The listing builds one solid part. Answer for the finished solid, in the listing's coordinates (mm). A direction names the side the tool comes from. Give positions to 0.01 mm unless a question says otherwise; leave off trailing zeros. Order: outer loops, then holes, each group sorted by start corner. A loop starts at its lowest first (then second) coordinate and runs counter-clockwise, first axis right, second up. Notation, with made-up numbers: (-21.5, 19.25) -> (15.5, 19.25) arc R34 ccw to (15.5, 51.25) -> close; hole circle Ø8 at (51, 15.25). An arc over 180 degrees is marked (long way). Answer as a JSON object with one key per item and string values. Group by question number.
Autodesk Inventor part; units mm, degrees
ref_plane "YZ Plane" through (0, 0, 0) normal (1, 0, 0) x (0, 1, 0)
ref_plane "XZ Plane" through (0, 0, 0) normal (0, 1, 0) x (-1, 0, 0)
ref_plane "XY Plane" through (0, 0, 0) normal (0, 0, 1) x (1, 0, 0)
sketch "Sketch1" plane through (0, 0, 0) normal (0, 1, 0) x (-1, 0, 0)
  line L0 (-7.5, 5.5) -> (7.5, 5.5)
  line L1 (7.5, 5.5) -> (7.5, -5.5)
  line L2 (7.5, -5.5) -> (-7.5, -5.5)
  line L3 (-7.5, -5.5) -> (-7.5, 5.5)
  line L4 (-7.5, 5.5) -> (7.5, -5.5) construction
  line L5 (7.5, 5.5) -> (-7.5, -5.5) construction
  circle A0 centre (0, -5.5) radius 7.5 construction
  arc A1 (-7.5, -5.5) -> (7.5, -5.5) centre (0, -5.5) ccw
  point P0 (0, 0)
  dimension "d0" = 11
  dimension "d1" = 15
extrude "Extrusion1" add sketch "Sketch1" along normal blind 8
sketch "Sketch2" plane through (0, 0, 0) normal (0, -1, 0) x (1, 0, 0)
  line L0 (7.5, 9.25) -> (-7.5, 9.25)
  line L1 (-7.5, 9.25) -> (-7.5, -20.75)
  line L2 (-7.5, -20.75) -> (7.5, -20.75)
  line L3 (7.5, -20.75) -> (7.5, 9.25)
  line L4 (7.5, 9.25) -> (-7.5, -20.75) construction
  line L5 (-7.5, 9.25) -> (7.5, -20.75) construction
  line L6 (-7.5, 5.5) -> (7.5, 5.5)
  line L7 (7, 8.75) -> (-7, 8.75) construction
  line L8 (-7, 8.75) -> (-7, -20.25) construction
  line L9 (-7, -20.25) -> (7, -20.25) construction
  line L10 (7, -20.25) -> (7, 8.75) construction
  line L11 (7, 8.75) -> (-7, -20.25) construction
  line L12 (-7, 8.75) -> (7, -20.25) construction
  point P0 (0, 0)
  point P1 (0, -5.75)
  dimension "d4" = 15
  dimension "d5" = 30
  dimension "d6" = 3.75
  dimension "d18" = 0.5
  dimension "d19" = 0.5
sketch "Sketch4" plane through (0, 0, 0) normal (0, -1, 0) x (1, 0, 0)
  line L0 (-7.5, -5.5) -> (-7.5, 5.5)
  line L1 (-7.5, 3.75) -> (-6.5, 3.75)
  line L2 (-6.5, 3.75) -> (-6.5, 0.75)
  line L3 (-6.5, 0.75) -> (-7.5, 0.75)
  line L4 (-7.5, 0.75) -> (-7.5, 3.75)
  line L5 (7.5, 5.5) -> (7.5, -5.5)
  line L6 (7.5, 0.75) -> (6.5, 0.75)
  line L7 (6.5, 0.75) -> (6.5, 3.75)
  line L8 (6.5, 3.75) -> (7.5, 3.75)
  line L9 (7.5, 3.75) -> (7.5, 0.75)
  line L10 (-7.5, -20.25) -> (7.5, -20.25) construction
  line L11 (7.5, -20.25) -> (7.5, 9.75) construction
  line L12 (7.5, 9.75) -> (-7.5, 9.75) construction
  line L13 (-7.5, 9.75) -> (-7.5, -20.25) construction
  line L14 (-7.5, -20.25) -> (7.5, 9.75) construction
  line L15 (7.5, -20.25) -> (-7.5, 9.75) construction
  line L16 (-7.5, 5.5) -> (7.5, 5.5) construction
  arc A0 (-7.5, -5.5) -> (7.5, -5.5) centre (0, -5.5) ccw construction
  point P0 (0, 0)
  point P1 (0, -5.25)
  point P2 (0, -13)
  point P3 (-7, 3.75)
  point P4 (-7.5, 0.75)
  point P5 (-7, 0.75)
  point P6 (7.5, 3.75)
  point P7 (-7.5, 0.75)
  dimension "d20" = 1
  dimension "d21" = 3
  dimension "d22" = 1
  dimension "d23" = 3
  dimension "d24" = 15
  dimension "d25" = 30
  dimension "d27" = 7.25
  dimension "d106" = 0.75
extrude "Extrusion3" add sketch "Sketch4" along normal blind 1.6
sketch "Sketch6" plane through (0, 0, 0) normal (0, -1, 0) x (1, 0, 0)
  line L0 (7.5, 11.25) -> (-7.5, 11.25)
  line L1 (-7.5, 11.25) -> (-7.5, -18.75)
  line L2 (-7.5, -18.75) -> (7.5, -18.75)
  line L3 (7.5, -18.75) -> (7.5, 11.25)
  line L4 (7.5, 11.25) -> (-7.5, -18.75) construction
  line L5 (-7.5, 11.25) -> (7.5, -18.75) construction
  line L6 (7, 10.75) -> (-7, 10.75) construction
  line L7 (-7, 10.75) -> (-7, -18.25) construction
  line L8 (-7, -18.25) -> (7, -18.25) construction
  line L9 (7, -18.25) -> (7, 10.75) construction
  line L10 (7, 10.75) -> (-7, -18.25) construction
  line L11 (-7, 10.75) -> (7, -18.25) construction
  circle A0 centre (0, -3.75) radius 1
  circle A1 centre (0, -3.75) radius 1.5
  line L12 (-6.5, 4.5) -> (6.5, 4.5)
  line L13 (6.5, 4.5) -> (6.5, -5.5)
  line L14 (6.5, -5.5) -> (-6.5, -5.5)
  line L15 (-6.5, -5.5) -> (-6.5, 4.5)
  line L16 (-7.5, 5.5) -> (7.5, 5.5)
  arc A2 (-7.5, -5.5) -> (7.5, -5.5) centre (0, -5.5) ccw
  circle A3 centre (0, -5.5) radius 6.5
  point P0 (0, 0)
  point P1 (-7.5, -3.75)
  point P2 (6.5, -5.5)
  dimension "d31" = 15
  dimension "d32" = 30
  dimension "d34" = 0.5
  dimension "d35" = 0.5
  dimension "d36" = 2
  dimension "d37" = 0.5
  dimension "d38" = 1
  dimension "d39" = 1
  dimension "d40" = 1
  dimension "d41" = 1
  dimension "d107" = 3.75
extrude "Extrusion4" cut sketch "Sketch6" against normal blind 2.5 contours A0 | L12 L13 A3 L15 | A3 L14 | L14 A3
sketch "Sketch10" plane through (0, 8, 0) normal (0, 1, 0) x (1, 0, 0)
  point P0 (0, 0)
sketch "Sketch11" plane through (0, 0, 0) normal (0, -1, 0) x (1, 0, 0)
  line L0 (-5, 3.5) -> (-2.5, 3.5)
  line L1 (-2.5, 3.5) -> (-2.5, 2)
  line L2 (-2.5, 2) -> (-5, 2)
  line L3 (-5, 2) -> (-5, 3.5)
  line L4 (2.5, 3.5) -> (5, 3.5)
  line L5 (5, 3.5) -> (5, 2)
  line L6 (5, 2) -> (2.5, 2)
  line L7 (2.5, 2) -> (2.5, 3.5)
  line L8 (-6.5, 3.75) -> (-7.5, 3.75)
  line L9 (-6.5, 0.75) -> (-6.5, 3.75)
  line L10 (6.5, 3.75) -> (6.5, 0.75)
  line L11 (-6.5, 4.5) -> (6.5, 4.5)
  line L12 (-1.25, -11) -> (1.25, -11)
  line L13 (1.25, -11) -> (1.25, -9.5)
  line L14 (1.25, -9.5) -> (-1.25, -9.5)
  line L15 (-1.25, -9.5) -> (-1.25, -11)
  circle A0 centre (0, -3.75) radius 1
  point P0 (0, 0)
  point P1 (-3.75, 3.5)
  point P2 (3.75, 3.5)
  point P3 (1.25, -10.25)
  point P4 (2.5, 2.75)
  point P5 (0, -9.5)
  point P6 (3.75, 2)
  point P7 (-2.5, 2.75)
  dimension "d51" = 2.5
  dimension "d52" = 1.5
  dimension "d55" = 2.75
  dimension "d56" = 2.75
  dimension "d60" = 13
  dimension "d61" = 3.75
  dimension "d62" = 3.75
  dimension "d103" = 6.5
  dimension "d104" = 6.5
extrude "Extrusion8" cut sketch "Sketch11" against normal blind 10 contours L0 L1 L2 L3 | L4 L5 L6 L7 | L15 L14 L13 L12
sketch "Sketch12" plane through (0, 2.5, 0) normal (0, -1, 0) x (1, 0, 0)
  line L0 (5, 2) -> (5, 3.5) construction
  line L1 (2.5, 2) -> (5, 2) construction
  line L2 (5, 3.5) -> (2.5, 3.5) construction
  line L3 (2.5, 3.5) -> (2.5, 2) construction
  line L4 (2.5, 2) -> (5, 2) construction
  line L5 (5, 2) -> (5, 3.5) construction
  line L6 (-2.5, 2) -> (-2.5, 3.5) construction
  line L7 (-2.5, 2) -> (-5, 2) construction
  line L8 (-2.5, 3.5) -> (-5, 3.5) construction
  line L9 (-5, 3.5) -> (-5, 2) construction
  line L10 (-5, 2) -> (-2.5, 2) construction
  line L11 (-2.5, 2) -> (-2.5, 3.5) construction
  line L12 (-1.25, -9.5) -> (1.25, -9.5) construction
  line L13 (-1.25, -9.5) -> (-1.25, -11) construction
  line L14 (1.25, -9.5) -> (-1.25, -9.5) construction
  line L15 (-1.25, -9.5) -> (-1.25, -11) construction
  line L16 (-1.25, -11) -> (1.25, -11) construction
  line L17 (1.25, -11) -> (1.25, -9.5) construction
  line L18 (5.5, 3.5) -> (2, 3.5)
  line L19 (2, 3.5) -> (2, 2)
  line L20 (2, 2) -> (5.5, 2)
  line L21 (5.5, 2) -> (5.5, 3.5)
  line L22 (1.75, -9.5) -> (-1.75, -9.5)
  line L23 (-1.75, -9.5) -> (-1.75, -11)
  line L24 (-1.75, -11) -> (1.75, -11)
  line L25 (1.75, -11) -> (1.75, -9.5)
  line L26 (-2, 3.5) -> (-5.5, 3.5)
  line L27 (-5.5, 3.5) -> (-5.5, 2)
  line L28 (-5.5, 2) -> (-2, 2)
  line L29 (-2, 2) -> (-2, 3.5)
  point P0 (0, 0)
  point P1 (-2.5, 2.75)
  point P2 (-2, 2.75)
  point P3 (-3.75, 2)
  point P4 (-3.75, 2)
  point P5 (-3.75, 3.5)
  point P6 (-3.75, 3.5)
  point P7 (-5, 2.75)
  point P8 (-5.5, 2.75)
  point P9 (1.25, -10.25)
  point P10 (1.75, -10.25)
  point P11 (0, -11)
  point P12 (-1.25, -10.25)
  dimension "d63" = 0.5
  dimension "d64" = 0
  dimension "d65" = 0
  dimension "d67" = 0.5
  dimension "d68" = 0
  dimension "d69" = 0
  dimension "d70" = 0.5
  dimension "d71" = 0.5
  dimension "d72" = 0
  dimension "d73" = 0
  dimension "d74" = 0.5
  dimension "d96" = 0.5
sketch "Sketch16" plane through (0, 2.5, 0) normal (0, -1, 0) x (1, 0, 0)
  line L0 (-6.5, -5.5) -> (-6.5, 4.5) construction
  line L1 (-6.5, 4.5) -> (6.5, 4.5) construction
  line L2 (-6.5, 4.5) -> (6.5, 4.5) construction
  line L3 (-0.5, 4.5) -> (0.5, 4.5)
  line L4 (0.5, 4.5) -> (0.5, -2.75)
  line L5 (0.5, -2.75) -> (-0.5, -2.75)
  line L6 (-0.5, -2.75) -> (-0.5, 4.5)
  circle A0 centre (0, -3.75) radius 1.5 construction
  circle A1 centre (0, -3.75) radius 1.75 construction
  line L7 (-6.5, -2.75) -> (6.5174, -2.75) construction
  circle A2 centre (0, -3.75) radius 1.5 construction
  circle A3 centre (0, -3.75) radius 1 construction
  line L8 (6.5, 0.75) -> (6.5, -5.5)
  line L9 (-6.5, -5.873) -> (6.5, -5.873)
  line L10 (6.5, -5.873) -> (6.5, -6.873)
  line L11 (6.5, -6.873) -> (-6.5, -6.873)
  line L12 (-6.5, -6.873) -> (-6.5, -5.873)
  point P0 (0, 0)
  point P1 (0, 4.5)
  point P2 (0.0087, -2.75)
  dimension "d94" = 1
  dimension "d95" = 1
extrude "Extrusion10" add sketch "Sketch16" along normal blind 2.5 contours L3 L4 L5 L6
sketch "Sketch18" plane through (0, 8, 0) normal (0, 1, 0) x (1, 0, 0)
  line L0 (0, 0) -> (0, 18.6084) construction
  circle A0 centre (0, 14) radius 1.5
  line L1 (-1.25, 11) -> (1.25, 11)
  dimension "d108" = 3
  dimension "d109" = 3
extrude "Extrusion12" add sketch "Sketch18" against normal blind 8
sketch "Sketch19" plane through (0, 2.5, -3.75) normal (0, -1, 0) x (1, 0, 0)
  circle A0 centre (0, 0) radius 1
  circle A1 centre (0, 0) radius 1
  point P0 (0, 3.75)
extrude "Extrusion13" cut sketch "Sketch19" against normal blind 4
sketch "Sketch14" plane through (0, 2.5, 0) normal (0, -1, 0) x (1, 0, 0)
  line L0 (5, 2.75) -> (2.5, 2.75) construction
  line L1 (2.5, 2.75) -> (2.5, 1.25) construction
  line L2 (2.5, 1.25) -> (5, 1.25) construction
  line L3 (5, 1.25) -> (5, 2.75) construction
  line L4 (5.5, 3.25) -> (2, 3.25)
  line L5 (2, 3.25) -> (2, 0.75)
  line L6 (2, 0.75) -> (5.5, 0.75)
  line L7 (5.5, 0.75) -> (5.5, 3.25)
  dimension "d86" = 0.5
  dimension "d87" = 0.5
sketch "Sketch15" plane through (0, 3.5, 0) normal (0, -1, 0) x (1, 0, 0)
  line L0 (5, 2.75) -> (2.5, 2.75)
  line L1 (2.5, 2.75) -> (2.5, 1.25)
  line L2 (2.5, 1.25) -> (5, 1.25)
  line L3 (5, 1.25) -> (5, 2.75)
  point P0 (0, 0)
sketch "Sketch8" plane through (0, 0, -3.75) normal (0, -1, 0) x (1, 0, 0)
  circle A0 centre (0, 0) radius 1.75
  circle A1 centre (0, 0) radius 1.5
  circle A2 centre (0, 0) radius 1.5
  point P0 (0, 3.75)
  dimension "d46" = 0.25
sketch "Sketch7" plane through (0, 2.5, -3.75) normal (0, -1, 0) x (1, 0, 0)
  circle A0 centre (0, 0) radius 1.25
  point P0 (0, 3.75)
properties part number "NANDGATE"
(1) Flat-ended cylindrical pins translate along their axes: pin 1 Ø2 at (y, z) = (0, -13) entering from +X; pin 2 Ø0.8 at (x, y) = (-7, -1) entering from +Z; pin 3 Ø5.5 at (x, z) = (-2, 0.5) entering from -Y. Find the tip coordinate at first contact, or state that the pin passes through.
(2) Find the intervals of material crossed by line 1 along Z through (x, y) = (0, 4.25); line 2 along X through (y, z) = (2, -3.75); line 3 along Z through (x, y) = (0, 1.5), in increasing order. Write a range as [from, to].
(3) Which of the six approach directions +Z, -Z, +X, -X, +Y, -Y give full straight-line access (tool end or side, diameter ignored) to faces 4 (the flat face through (2.5, 5, 3)), 5 (the flat face through (-4, 1, 4.5)), 6 (the flat face through (7.5, 4, 0)), 7 (the flat face through (7, -1, 3.75)), 8 (the flat face through (-7, -1.6, 2))?
(4) For a pull along Z with two mould halves and no side action, classify faces 1 (the flat face through (-7, -1, 0.75)), 2 (the flat face through (7, -1.6, 2)), 3 (the flat face through (0, 6.5, -4)) as +Z half, -Z half, draft (parallel to the pull), parting line (faces both ways), or undercut.
(5) A cutting plane is placed at D-D (y = 6). Determine the outline of the cut face in (x, z).
(6) A cutting plane is placed at C-C (z = -0.5). Determine the outline of the cut face in (x, y).
(7) A cutting plane is placed at B-B (x = 0). Determine the outline of the cut face in (y, z).
(8) A cutting plane is placed at A-A (y = -0.25). Determine the outline of the cut face in (x, z), and give its area (3 significant figures).
Check sheet entries:
{
 "1": {"pin 1": "stops at x = 3.74", "pin 2": "stops at z = 3.75", "pin 3": "stops at y = 0"},
 "2": {"line 1": "z = [-15.5, -11], [-9.5, -4.75], [-2.75, 5.5]", "line 2": "x = [-7.5, -6.5], [-1.5, -1], [1, 1.5], [6.5, 7.5]", "line 3": "z = [-15.5, -12], [-5.25, -4.75], [-2.75, 5.5]"},
 "3": {"face 4": "+Y, -Y", "face 5": "-Y", "face 6": "+Z, -Z, +X, +Y, -Y", "face 7": "+Z, +X, -X, -Y", "face 8": "+Z, -Z, +X, -X, -Y"},
 "4": {"face 1": "-Z half", "face 2": "draft", "face 3": "undercut"},
 "5": {"outline": "(-7.5, -5.5) arc R7.5 ccw to (-1.05, -12.93) arc R1.5 ccw (long way) to (1.05, -12.93) arc R7.5 ccw to (7.5, -5.5) -> (7.5, 5.5) -> (-7.5, 5.5) -> close; hole (-5, 2) -> (-2.5, 2) -> (-2.5, 3.5) -> (-5, 3.5) -> close; hole (-1.25, -11) -> (1.25, -11) -> (1.25, -9.5) -> (-1.25, -9.5) -> close; hole circle Ø2 at (0, -3.75); hole (2.5, 2) -> (5, 2) -> (5, 3.5) -> (2.5, 3.5) -> close"},
 "6": {"outline": "(-7.5, 0) -> (-6.5, 0) -> (-6.5, 2.5) -> (-0.5, 2.5) -> (-0.5, 0) -> (0.5, 0) -> (0.5, 2.5) -> (6.5, 2.5) -> (6.5, 0) -> (7.5, 0) -> (7.5, 8) -> (-7.5, 8) -> close"},
 "7": {"outline": "(0, -15.5) -> (8, -15.5) -> (8, -11) -> (2.5, -11) -> (2.5, -12) -> (0, -12) -> close; (0, -5.25) -> (2.5, -5.25) -> (2.5, -9.5) -> (8, -9.5) -> (8, 5.5) -> (0, 5.5) -> (0, -2.75) -> (6.5, -2.75) -> (6.5, -4.75) -> (0, -4.75) -> close"},
 "8": {"outline": "(-7.5, 0.75) -> (-6.5, 0.75) -> (-6.5, 3.75) -> (-7.5, 3.75) -> close; (6.5, 0.75) -> (7.5, 0.75) -> (7.5, 3.75) -> (6.5, 3.75) -> close", "area": "6.00 mm2"}
}
